from build123d import *

# Parameters (mm, degrees)
F0_W        = 10
F0_H        = 20
F1_DEPTH    = 10
F3_DEPTH    = 5
F4_T4_DEPTH = 35.7168298797
F4_T9_DEPTH = 35.7168298797
F5_SIZE     = 2
F7_DEPTH    = 26
F9_DEPTH    = 10
F9_TAPER    = -10
F11_DEPTH   = 5
F12_DEPTH   = 9
F13_R       = 1
F14_W       = 4
F14_H       = 8
F15_DEPTH   = 1
F16_SIZE    = 0.99999
F17_DEPTH   = 5


# Not quite as in the source:
# - a fillet or chamfer that OpenCascade refuses, or shapes differently, is made with other operations: its cross-section is extruded or revolved along the edge and cut away or added
# - a fillet or chamfer is up to 0.001 mm smaller than in the source, because OpenCascade refuses the exact size
# - a feature names something its author has since deleted; it is built from what else it names


with BuildPart() as f1:
    # F0 (on Top) → F1 (new body)
    with BuildSketch(Plane.XY):
        with Locations((-7.7272727273, 0)):
            Rectangle(F0_W, F0_H)
        Polygon((-2.7272727273, 13), (-2.7272727273, 10), (-2.7272727273, -10), (-2.7272727273, -13), (27.2727272727, -13), (27.2727272727, 13), align=None)
    extrude(amount=F1_DEPTH)

    # F2 (on face) → F3 (cut)
    with BuildSketch(Plane(origin=(-12.7272727273, 0, 0), x_dir=(0, -1, 0), z_dir=(-1, 0, 0))):
        Polygon((0, 5), (-2.7, 6.35), (-5.35, 6.35), (-5.35, 3.65), (-2.7, 3.65), align=None)
        Polygon((2.7, 3.65), (0, 5), (-2.7, 3.65), align=None)
        Polygon((2.7, 6.35), (0, 5), (2.7, 3.65), (5.35, 3.65), (5.35, 6.35), align=None)
        Polygon((2.7, 6.35), (-2.7, 6.35), (0, 5), align=None)
    extrude(amount=-F3_DEPTH, mode=Mode.SUBTRACT)

    # F4: chamfer of 5 on 2 edges, made by hand


with BuildPart() as f4_tool2:
    # F4_s3 → F4_t4 (new body)
    with BuildSketch(Plane.XY.offset(-12.8584149398)):
        Polygon((2.2727272727, 13), (-2.7272727273, 8), (-2.7272727273, 13), align=None)
    extrude(amount=F4_T4_DEPTH)

    split(bisect_by=Plane.XZ.offset(-10), keep=Keep.BOTTOM)


with BuildPart() as f1_1:
    add(f1.part)

    # F4_t1: cut F4_tool2
    add(f4_tool2.part, mode=Mode.SUBTRACT)


with BuildPart() as f4_tool7:
    # F4_s8 → F4_t9 (new body)
    with BuildSketch(Plane.XY.offset(-12.8584149398)):
        Polygon((-2.7272727273, -8), (2.2727272727, -13), (-2.7272727273, -13), align=None)
    extrude(amount=F4_T9_DEPTH)

    split(bisect_by=Plane.XZ.offset(10), keep=Keep.TOP)


with BuildPart() as f1_2:
    add(f1_1.part)

    # F4_t6: cut F4_tool7
    add(f4_tool7.part, mode=Mode.SUBTRACT)

    # F5
    f5_edges = [f1_2.edges().sort_by_distance(p)[0] for p in [
        (-12.727273, 10, 5),
        (-12.727273, -10, 5),
    ]]
    chamfer(f5_edges, length=F5_SIZE)

    # F6 (on face) → F7 (cut, through all)
    with BuildSketch(Plane(origin=(0, 13, 0), x_dir=(-1, 0, 0), z_dir=(0, 1, 0))):
        Polygon((-14.7727272727, 5), (-17.2727272727, 6), (-17.2727272727, 5), align=None)
        Polygon((-17.2727272727, 6.45), (-17.2727272727, 6), (-14.7727272727, 5), (-11.1477272727, 6.45), align=None)
        Polygon((-11.1477272727, 6.45), (-14.7727272727, 5), (-6.3727272727, 5), (-6.3727272727, 6.45), align=None)
        Polygon((-17.2727272727, 4), (-14.7727272727, 5), (-17.2727272727, 5), align=None)
        Polygon((-11.1477272727, 3.55), (-14.7727272727, 5), (-17.2727272727, 4), (-17.2727272727, 3.55), align=None)
        Polygon((-6.3727272727, 5), (-14.7727272727, 5), (-11.1477272727, 3.55), (-6.3727272727, 3.55), align=None)
    extrude(amount=-F7_DEPTH, mode=Mode.SUBTRACT)

    # F8 (on face) → F9 (cut, through all)
    with BuildSketch(Plane.YZ.offset(27.2727272727)):
        with BuildLine():
            Line((-2.4, 5), (0, 5))
            Line((0, 5), (-2.2400294549, 5.8615497903))
            ThreePointArc((-2.2400294549, 5.8615497903), (-2.3596684822, 5.4381377114), (-2.4, 5))
        make_face()
        with BuildLine():
            Line((-2.2400294549, 5.8615497903), (0, 5))
            Line((0, 5), (2.2400294549, 5.8615497903))
            ThreePointArc((2.2400294549, 5.8615497903), (0, 7.4), (-2.2400294549, 5.8615497903))
        make_face()
        with BuildLine():
            Line((0, 5), (2.2400294549, 4.1384502097))
            ThreePointArc((2.2400294549, 4.1384502097), (2.3596684822, 4.5618622886), (2.4, 5))
            ThreePointArc((2.4, 5), (2.3596684822, 5.4381377114), (2.2400294549, 5.8615497903))
            Line((2.2400294549, 5.8615497903), (0, 5))
        make_face()
        with BuildLine():
            ThreePointArc((-2.2400294549, 4.1384502097), (0, 2.6), (2.2400294549, 4.1384502097))
            Line((2.2400294549, 4.1384502097), (0, 5))
            Line((0, 5), (-2.2400294549, 4.1384502097))
        make_face()
        with BuildLine():
            Line((-2.2400294549, 4.1384502097), (0, 5))
            Line((0, 5), (-2.4, 5))
            ThreePointArc((-2.4, 5), (-2.3596684822, 4.5618622886), (-2.2400294549, 4.1384502097))
        make_face()
    extrude(amount=-F9_DEPTH, taper=F9_TAPER, mode=Mode.SUBTRACT)

    # F10 (on face) → F11 (cut)
    with BuildSketch(Plane(origin=(0, 0, 0), x_dir=(1, 0, 0), z_dir=(0, 0, -1))):
        Polygon((18.2727272727, -3), (18.2727272727, 3), (16.2727272727, 3), (8.2727272727, 3), (8.2727272727, -3), (16.2727272727, -3), align=None)
    extrude(amount=-F11_DEPTH, mode=Mode.SUBTRACT)

    # F12 (cut, through all): faces of the model
    f12_faces = [f1_2.faces().sort_by_distance(p)[0] for p in [
        (17.2727272727, 3.3247194786, 3.0369278497),
        (17.2727272727, -3.3247194786, 3.0369278497),
    ]]
    extrude(f12_faces, amount=-F12_DEPTH, mode=Mode.SUBTRACT)

    # F13
    f13_edges = [f1_2.edges().sort_by_distance(p)[0] for p in [
        (18.272727, -3, 1.187016),
        (8.272727, -3, 1.056669),
        (8.272727, 3, 1.056669),
        (18.272727, 3, 1.187016),
    ]]
    fillet(f13_edges, radius=F13_R)

    # F14 (on face) → F15 (cut)
    with BuildSketch(Plane(origin=(0, 0, 0), x_dir=(1, 0, 0), z_dir=(0, 0, -1))):
        Polygon((8.2727272727, 2), (-12.7272727273, 2), (-12.7272727273, -2), (-6.7272727273, -2), (-2.7272727273, -2), (8.2727272727, -2), align=None)
        with Locations((-4.7272727273, -6)):
            Rectangle(F14_W, F14_H)
    extrude(amount=-F15_DEPTH, mode=Mode.SUBTRACT)

    # F16 (size 1 in the source; OpenCascade refuses exactly that, so slightly less here)
    f16_edges = [f1_2.edges().sort_by_distance(p)[0] for p in [
        (-6.727273, 6, 0),
    ]]
    chamfer(f16_edges, length=F16_SIZE)

    # F8 (on face) → F17 (cut)
    with BuildSketch(Plane.YZ.offset(27.2727272727)):
        Polygon((-4, 7.5), (-6.5, 7.5), (-4, 6.5384615385), align=None)
        Polygon((-4, 6.5384615385), (-6.5, 7.5), (-9, 7.5), (-9, 5), (-4, 5), align=None)
        Polygon((-9, 2.5), (-6.5, 2.5), (-4, 3.4615384615), (-4, 5), (-9, 5), align=None)
        Polygon((-4, 3.4615384615), (-6.5, 2.5), (-4, 2.5), align=None)
    extrude(amount=-F17_DEPTH, mode=Mode.SUBTRACT)


solid = f1_2.part
Work out the finished part from the listing and answer in its coordinate system (mm). A direction names the side the tool comes from. Give positions to 0.01 mm unless a question says otherwise; leave off trailing zeros. Order: outer loops, then holes, each group sorted by start corner. A loop starts at its lowest first (then second) coordinate and runs counter-clockwise, first axis right, second up. Notation, with made-up numbers: M 37.5,64.25 L 53.5,64.25 A32 ccw 53.5,91.25 Z; hole C 69.25,-1.75 d7. An arc over 180 degrees is marked long. Return JSON: item names as keys, results as strings.
Q1. The mould has two halves that part along Y. Classify faces 5 (the face through (-11.713, 9.014, 4.93)), 6 (the face through (6.373, 0, 5)), 7 (the face through (-11.713, -9.014, 4.93)), 8 (the face through (17.972, 2.715, 1.087)): pulls with the +Y half, pulls with the -Y half, needs draft (parallel to the pull), parting line crosses it, or undercut.
Answer below:
{"face 5": "pulls with the +Y half", "face 6": "needs draft", "face 7": "pulls with the -Y half", "face 8": "undercut"}
Q2. Find the intervals of material crossed by line 1 along Y through (x, z) = (16, 1); line 2 along Y through (x, z) = (24.5, 6.5); line 3 along Z through (x, y) = (16, -6.5), in increasing order. Write a range as [from, to].
Answer below:
{"line 1": "y = [-13, -3], [3, 13]", "line 2": "y = [-13, -9], [-4, -2.47], [2.47, 13]", "line 3": "z = [0, 3.55], [6.45, 10]"}
Q3. Which of the six approach directions +Z, -Z, +X, -X, +Y, -Y give full straight-line access (tool end or side, diameter ignored) to faces 1 (the face through (-10, -5.35, 5)), 2 (the face through (25, -7, 2.5)), 3 (the face through (8, 0, 3.55)), 4 (the face through (13, 3, 1))?
Answer below:
{"face 1": "-X", "face 2": "+X", "face 3": "+Y, -Y", "face 4": "-Z"}
Q4. Find section B-B, the plane x = 12. Write down the section's boundary in (y, z), and give its area (3 significant figures).
Answer below:
{"outline": "M -13,0 L -3,0 L -3,2.11 A4.16 cw -3.9,3.55 L -13,3.55 Z; M -13,6.45 L 13,6.45 L 13,10 L -13,10 Z; M 3,0 L 13,0 L 13,3.55 L 3.9,3.55 A4.16 cw 3,2.11 Z", "area": "162 mm^2"}
Q5. Each of these flat-tipped pins is pushed along its axis until it touches: pin 1 (2.5 mm diameter, centred on y = -10, z = 5, fed in from -X); pin 2 (1.5 mm diameter, centred on x = -6.5, y = 6.5, fed in from -Z); pin 3 (0.8 mm diameter, centred on x = -11, z = 5, fed in from -Y). Where does it stop, or does it pass through?
Answer below:
{"pin 1": "stops at x = -11.98", "pin 2": "stops at z = 0.48", "pin 3": "stops at y = -10"}
Q6. Find section C-C, the plane x = -6. Write down the section's boundary in (y, z), and give its area (3 significant figures).
Answer below:
{"outline": "M -10,0 L -2,0 L -2,1 L 10,1 L 10,10 L -10,10 Z", "area": "188 mm^2"}
Q7. Find section D-D, the plane x = 25. State how many separate pieces and enclosed holes the cut face has, and give its area (3 significant figures).
Answer below:
{"separate pieces": "1", "enclosed holes": "2", "area": "210 mm^2"}
